from build123d import *

# Parameters (mm, degrees)
SKETCH1_W           = 40
SKETCH1_H           = 30
BOSS_EXTRUDE1_DEPTH = 15
SKETCH2_W           = 20
SKETCH2_H           = 4
BOSS_EXTRUDE2_DEPTH = 11
SKETCH3_R           = 1.5
CUT_EXTRUDE1_DEPTH  = 20
SKETCH4_W           = 4
SKETCH4_H           = 6
BOSS_EXTRUDE3_DEPTH = 5
CUT_EXTRUDE2_DEPTH  = 21
FILLET7_R           = 6
FILLET8_R           = 6
FILLET9_R           = 6
FILLET10_R          = 6
CUT_EXTRUDE5_START  = -40
CUT_EXTRUDE5_DEPTH  = 40


# Read off the part's stored shape, not the designer's step: Cut-Extrude5
with BuildPart() as part:
    # Sketch1 → Boss-Extrude1 (new body)
    with BuildSketch(Plane(origin=(0, 0, 0), x_dir=(1, 0, 0), z_dir=(0, 1, 0))):
        with Locations((20, 15)):
            Rectangle(SKETCH1_W, SKETCH1_H)
    extrude(amount=BOSS_EXTRUDE1_DEPTH)

    # Sketch2 → Boss-Extrude2 (add)
    with BuildSketch(Plane(origin=(0, 15, 0), x_dir=(1, 0, 0), z_dir=(0, 1, 0))):
        with Locations((20, 22)):
            Rectangle(SKETCH2_W, SKETCH2_H)
        with Locations((20, 8)):
            Rectangle(SKETCH2_W, SKETCH2_H)
    extrude(amount=BOSS_EXTRUDE2_DEPTH)

    # Sketch3 → Cut-Extrude1 (cut)
    with BuildSketch(Plane.XY.offset(-6)):
        with BuildLine():
            Line((10, 26), (10, 19.638135164))
            ThreePointArc((10, 19.638135164), (13.769016564, 24.093247122), (19.284250184, 26))
            Line((19.284250184, 26), (10, 26))
        make_face()
        with BuildLine():
            Line((30, 26), (20.715749816, 26))
            ThreePointArc((20.715749816, 26), (26.230983436, 24.093247122), (30, 19.638135164))
            Line((30, 19.638135164), (30, 26))
        make_face()
        with Locations((20, 20.5)):
            Circle(SKETCH3_R)
    extrude(amount=-CUT_EXTRUDE1_DEPTH, mode=Mode.SUBTRACT)

    # Sketch4 → Boss-Extrude3 (add)
    with BuildSketch(Plane(origin=(0, 15, 0), x_dir=(1, 0, 0), z_dir=(0, 1, 0))):
        with Locations((14, 27)):
            Rectangle(SKETCH4_W, SKETCH4_H)
        with Locations((26, 27)):
            Rectangle(SKETCH4_W, SKETCH4_H)
        with Locations((14, 3)):
            Rectangle(SKETCH4_W, SKETCH4_H)
        with Locations((26, 3)):
            Rectangle(SKETCH4_W, SKETCH4_H)
    extrude(amount=BOSS_EXTRUDE3_DEPTH)

    # Sketch5 → Cut-Extrude2 (cut)
    with BuildSketch(Plane(origin=(28, 0, 0), x_dir=(0, 0, -1), z_dir=(1, 0, 0))):
        Polygon((0, 15), (0, 20), (6, 20), align=None)
        Polygon((24, 20), (30, 20), (30, 15), align=None)
    extrude(amount=-CUT_EXTRUDE2_DEPTH, mode=Mode.SUBTRACT)

    # Fillet7
    fillet7_edges = [part.edges().sort_by_distance(p)[0] for p in [
        (0, 7.5, 0),
    ]]
    fillet(fillet7_edges, radius=FILLET7_R)

    # Fillet8
    fillet8_edges = [part.edges().sort_by_distance(p)[0] for p in [
        (0, 7.5, -30),
    ]]
    fillet(fillet8_edges, radius=FILLET8_R)

    # Fillet9
    fillet9_edges = [part.edges().sort_by_distance(p)[0] for p in [
        (40, 7.5, -30),
    ]]
    fillet(fillet9_edges, radius=FILLET9_R)

    # Fillet10
    fillet10_edges = [part.edges().sort_by_distance(p)[0] for p in [
        (40, 7.5, 0),
    ]]
    fillet(fillet10_edges, radius=FILLET10_R)

    # Cut-Extrude5 outline → Cut-Extrude5 (cut)
    with BuildSketch(Plane.ZY.offset(CUT_EXTRUDE5_START)):
        with BuildLine():
            ThreePointArc((-0.15376037, 1.624355142), (-1.070457114, 0.445844195), (-2.495393579, 0))
            Line((-2.495393579, 0), (0, 0))
            Line((0, 0), (0, 1.624355142))
            Line((0, 1.624355142), (-0.15376037, 1.624355142))
        make_face()
        with BuildLine():
            Line((-30, 0), (-27.499999999, 0))
            ThreePointArc((-27.499999999, 0), (-28.924936464, 0.445844194), (-29.841633208, 1.624355142))
            Line((-29.841633208, 1.624355142), (-30, 1.624355142))
            Line((-30, 1.624355142), (-30, 0))
        make_face()
        with BuildLine():
            Line((-27.499999999, 0), (-22.499999999, 0))
            ThreePointArc((-22.499999999, 0), (-23.924936464, 0.445844194), (-24.841633208, 1.624355142))
            Line((-24.841633208, 1.624355142), (-25.158366792, 1.624355142))
            ThreePointArc((-25.158366792, 1.624355142), (-26.075063535, 0.445844195), (-27.499999999, 0))
        make_face()
        with BuildLine():
            Line((-22.499999999, 0), (-17.5, 0))
            ThreePointArc((-17.5, 0), (-18.924936464, 0.445844195), (-19.841633208, 1.624355142))
            Line((-19.841633208, 1.624355142), (-20.158366792, 1.624355142))
            ThreePointArc((-20.158366792, 1.624355142), (-21.075063535, 0.445844195), (-22.499999999, 0))
        make_face()
        with BuildLine():
            Line((-17.5, 0), (-12.446445217, 0))
            ThreePointArc((-12.446445217, 0), (-13.871381681, 0.445844195), (-14.788078425, 1.624355142))
            Line((-14.788078425, 1.624355142), (-15.158366792, 1.624355142))
            ThreePointArc((-15.158366792, 1.624355142), (-16.075063536, 0.445844195), (-17.5, 0))
        make_face()
        with BuildLine():
            Line((-12.446445217, 0), (-7.490821514, 0))
            ThreePointArc((-7.490821514, 0), (-8.91575797, 0.445844198), (-9.832454709, 1.624355142))
            Line((-9.832454709, 1.624355142), (-10.104812008, 1.624355142))
            ThreePointArc((-10.104812008, 1.624355142), (-11.021508752, 0.445844195), (-12.446445217, 0))
        make_face()
        with BuildLine():
            ThreePointArc((-2.495393579, 0), (-3.920330043, 0.445844195), (-4.837026787, 1.624355142))
            Line((-4.837026787, 1.624355142), (-5.149188292, 1.624355142))
            ThreePointArc((-5.149188292, 1.624355142), (-6.065885042, 0.445844191), (-7.490821514, 0))
            Line((-7.490821514, 0), (-2.495393579, 0))
        make_face()
    extrude(amount=CUT_EXTRUDE5_DEPTH, mode=Mode.SUBTRACT)


solid = part.part
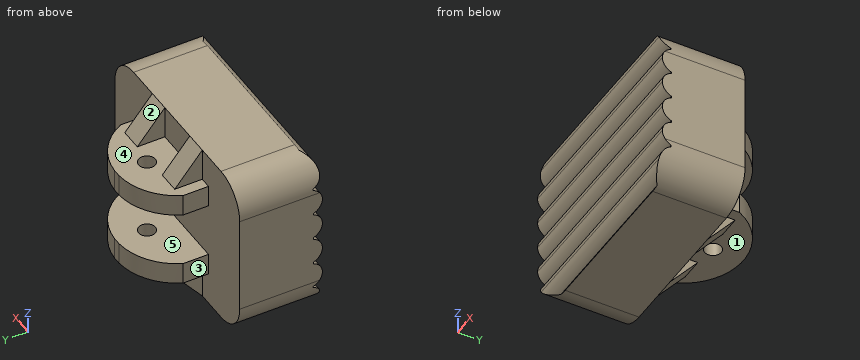
Read the model definition and answer for the solid it produces. Units are mm, in the model's axes. Face numbers are marked on the shaded views. A direction names the side the tool comes from. Give positions to 0.01 mm unless a question says otherwise; leave off trailing zeros. Write each loop counter-clockwise with the first axis right and the second up, starting at its lowest first coordinate (ties: lowest second). Pieces come first, ordered by that corner, then holes. Notation, with made-up numbers: (72.25, -28) - (106.25, -28) arc R15 cw to (106.25, 1) - close; hole circle Ø11 at (-33.5, -27.5). An arc over 180 degrees is marked (long way). Answer in a Markdown table with one row per item. Add a question column.
Item 1: Section B-B, the plane y = 20.5 is taken. Write down the section's boundary in (x, z), and give its area (3 significant figures).
Item 2: Flat-ended cylindrical pins translate along their axes: P1, Ø5, axis at x = 20, y = 20.5, coming from the -Z side; P2, Ø1, axis at x = 24, z = -23.5, coming from the -Y side; P3, Ø5, axis at y = 20, z = -23.5, coming from the +X side. Find the tip coordinate at first contact, or state that the pin passes through.
Item 3: A tool of negligible diameter and unlimited length cuts with its end or side. For the marked faces 1, 2, 3, 4 and 5, from which of +Z, -Z, +X, -X, +Y, -Y can it reach the whole face along a straight path? Write none if from no direction.
Item 4: Find the intervals of material crossed by L1, parallel to Z at x = 17, y = 18.75; L2, parallel to Y at x = 2, z = -7; L3, parallel to Y at x = 20, z = -8.4, in increasing order.
Item 5: Section D-D, the plane x = 20 is taken. Count the separate pieces of the cut face and the enclosed holes in it, and give its area (3 significant figures).
Item 6: Section C-C, the plane y = 6.5 is taken. Write down the section's boundary in (x, z), and give its area (3 significant figures).
Item 7: Section A-A, the plane x = 30.5 is taken. Write down the section's boundary in (y, z).
Recorded:
| question | item | result |
|---|---|---|
| 1 | outline | (10.45, -24) - (18.5, -24) - (18.5, -20) - (10.45, -20) - close; (10.45, -10) - (18.5, -10) - (18.5, -6) - (10.45, -6) - close; (21.5, -24) - (29.55, -24) - (29.55, -20) - (21.5, -20) - close; (21.5, -10) - (29.55, -10) - (29.55, -6) - (21.5, -6) - close |
| 1 | area | 129 mm2 |
| 2 | P1 | stops at z = -24 |
| 2 | P2 | stops at y = 0.05 |
| 2 | P3 | stops at x = 30 |
| 3 | face 1 | -Z, +Y |
| 3 | face 2 | +Z, +X, -X, +Y |
| 3 | face 3 | +Z, -Z, -X, +Y |
| 3 | face 4 | +Z, +Y |
| 3 | face 5 | +X, -X, +Y |
| 4 | L1 | z = -24 to -20, -10 to -6 |
| 4 | L2 | y = 0.05 to 15 |
| 4 | L3 | y = 0.17 to 19, 22 to 26 |
| 5 | separate pieces | 3 |
| 5 | enclosed holes | 0 |
| 5 | area | 498 mm2 |
| 6 | outline | (0, -24) arc R6 ccw to (6, -30) - (34, -30) arc R6 ccw to (40, -24) - (40, -6) arc R6 ccw to (34, 0) - (6, 0) arc R6 ccw to (0, -6) - close |
| 6 | area | 1,170 mm2 |
| 7 | outline | (1.62, -30) - (15, -30) - (15, 0) - (1.62, 0) - (1.62, -0.15) arc R2.5 ccw to (1.62, -4.84) - (1.62, -5.15) arc R2.5 ccw to (1.62, -9.83) - (1.62, -10.1) arc R2.5 ccw to (1.62, -14.79) - (1.62, -15.16) arc R2.5 ccw to (1.62, -19.84) - (1.62, -20.16) arc R2.5 ccw to (1.62, -24.84) - (1.62, -25.16) arc R2.5 ccw to (1.62, -29.84) - close |
